Read the model definition and answer for the solid it produces. Units are mm, in the model's axes. A direction names the side the tool comes from. Coordinates: 2 decimals unless noted, no trailing zeros. Write each loop counter-clockwise with the first axis right and the second up, starting at its lowest first coordinate (ties: lowest second). Pieces come first, ordered by that corner, then holes. Notation, with made-up numbers: (-27.5, 51) - (17.5, 51) arc R14 cw to (17.5, 60) - close; hole circle Ø6 at (64.5, 43). An arc over 180 degrees is marked (long way). Return JSON: item names as keys, results as strings.
```python
from build123d import *

# Parameters (mm, degrees)
SKETCH1_W           = 50
SKETCH1_H           = 35
BOSS_EXTRUDE1_DEPTH = 2.6
CAVITY1_OUTLINE_W   = 47.4
CAVITY1_OUTLINE_H   = 2.6
CAVITY1_DEPTH       = 2.6


# Read off the part's stored shape, not the designer's step: Cavity1
with BuildPart() as part:
    # Sketch1 → Boss-Extrude1 (new body)
    with BuildSketch(Plane.XY):
        with Locations((25, 17.5)):
            Rectangle(SKETCH1_W, SKETCH1_H)
    extrude(amount=BOSS_EXTRUDE1_DEPTH)

    # Cavity1 outline → Cavity1 (cut)
    with BuildSketch(Plane(origin=(0, 0, 0), x_dir=(1, 0, 0), z_dir=(0, 1, 0))):
        with Locations((26.3, -1.3)):
            Rectangle(CAVITY1_OUTLINE_W, CAVITY1_OUTLINE_H)
    extrude(amount=CAVITY1_DEPTH, mode=Mode.SUBTRACT)


solid = part.part
```
(1) A straight line is drawn through the part: line 1 (Y direction, x = 28.5, z = 0.9). Find the intervals that lie inside material, in ascending order. Write a range as from..to.
Answer:
{"line 1": "2.6..35"}
(2) A cutting plane is placed at B-B (x = 8.5). Determine the outline of the cut face in (y, z).
Answer:
{"outline": "(2.6, 0) - (35, 0) - (35, 2.6) - (2.6, 2.6) - close"}
(3) Which of the six approach directions +Z, -Z, +X, -X, +Y, -Y give full straight-line access (tool end or side, diameter ignored) to faces 1 (the face through (2.6, 1, 1)), 2 (the face through (1, 0, 1))?
Answer:
{"face 1": "+Z, -Z, +X, -Y", "face 2": "+Z, -Z, +X, -X, -Y"}
(4) A cutting plane is placed at A-A (z = 0.65). Determine the outline of the cut face in (x, y), and give its area (3 significant figures).
Answer:
{"outline": "(0, 0) - (2.6, 0) - (2.6, 2.6) - (50, 2.6) - (50, 35) - (0, 35) - close", "area": "1,630 mm²"}
(5) A flat-ended cylindrical pin translates along its axis: P1, Ø1.3, axis at x = 32.5, z = 2, coming from the -Y side. Find the tip coordinate at first contact, or state that the pin passes through.
Answer:
{"P1": "y = 2.6"}
